```python
from build123d import *

# Parameters (mm, degrees)
SKETCH1_R           = 1.675263483
SKETCH1_R_2         = 0.75
BOSS_EXTRUDE1_DEPTH = 10
SKETCH3_W           = 0.497124842
SKETCH3_H           = 1


with BuildPart() as part:
    # Sketch1 → Boss-Extrude1 (new body, symmetric)
    with BuildSketch(Plane.XY):
        with Locations((-12.495417101, 27.339793711)):
            Circle(SKETCH1_R)
        with Locations((-12.495417101, 27.339793711)):
            Circle(SKETCH1_R_2, mode=Mode.SUBTRACT)
    extrude(amount=BOSS_EXTRUDE1_DEPTH, both=True)

    # Sweep1: sweep along a path in Sketch2
    with BuildLine(Plane.XY) as sweep1_path:
        ThreePointArc((-12.495417101, 27.339793711), (60.808757123, 5.185065564), (-12.495417101, -16.969662583))
    # Sketch3 → Sweep1 (sweep)
    with BuildSketch(Plane(origin=(-12.495417101, 27.339793711, 0), x_dir=(0, 0, 1), z_dir=(0.553868204, 0.832604356, 0))):
        Rectangle(SKETCH3_W, SKETCH3_H)
    sweep(path=sweep1_path.line)


solid = part.part
```
Check sheet for the modelled part. Datum: model origin and axes. Units: mm. Coordinates: 2 decimals unless noted, no trailing zeros. Loops run counter-clockwise (first coordinate to the right, second up) from the corner with the lowest first, then second, coordinate; pieces in that order, holes last.
1) Material ranges on probe 1 along Y at (x, z) = (-8.5, 0); probe 2 along X at (y, z) = (28, -2.5); probe 3 along X at (y, z) = (9, 0), recorded low to high.
2) Sectioned sample at B-B (y = 40.5). Record the boundary of the cut face in (x, z).
3) Gauge pin test, flat ends, axial feed: pin 1 (1.4 mm diameter, centred on x = -12.5, y = 27.34, fed in from +Z); pin 2 (22.5 mm diameter, centred on x = 40.5, y = -13.5, fed in from -Z); pin 3 (8 mm diameter, centred on y = 31.5, z = 8, fed in from -X); pin 4 (10 mm diameter, centred on x = -4, z = 2.5, fed in from +Y). Record the tip position at first contact, or that the pin passes through.
4) Sectioned sample at C-C (y = 17.5). Record the boundary of the cut face in (x, z), and give its area (3 significant figures).
5) Release check for a two-part mould opening along Y. For faces 1 (the face through (60.304, 5.792, -0.003)), 2 (the face through (60, -4, 0.249)), 3 (the face through (61.304, 5.818, 0.003)) record: released by +Y, released by -Y, zero draft, split by the parting line, or undercut.
6) Sectioned sample at A-A (x = 31). Record the boundary of the cut face in (y, z).
7) Sectioned sample at D-D (z = 8.5). Record the boundary of the cut face in (x, y), and give its area (3 significant figures).
Check sheet entries:
1. probe 1: y = -22.77 to -21.3, 31.67 to 33.14
1. probe 2: x = -14.04 to -12.85, -12.14 to -10.96
1. probe 3: x = 60.12 to 61.13
2. outline: (0.98, -0.25) - (3.11, -0.25) - (3.11, 0.25) - (0.98, 0.25) - close; (38.5, -0.25) - (40.64, -0.25) - (40.64, 0.25) - (38.5, 0.25) - close
3. pin 1: stops at z = 0.25
3. pin 2: passes through
3. pin 3: stops at x = -14.16
3. pin 4: stops at y = 40.2
4. outline: (58.34, -0.25) - (59.39, -0.25) - (59.39, 0.25) - (58.34, 0.25) - close
4. area: 0.523 mm2
5. face 1: undercut
5. face 2: zero draft
5. face 3: split by the parting line
6. outline: (-34.01, -0.25) - (-32.98, -0.25) - (-32.98, 0.25) - (-34.01, 0.25) - close; (43.35, -0.25) - (44.38, -0.25) - (44.38, 0.25) - (43.35, 0.25) - close
7. outline: circle Ø3.35 at (-12.5, 27.34); hole circle Ø1.5 at (-12.5, 27.34)
7. area: 7.05 mm2
